For this review, take the finished solid that the model builds, in its own axes (mm). Face numbers are marked on the shaded views. A direction names the side the tool comes from. Give positions to 0.01 mm unless a question says otherwise; leave off trailing zeros. Loops run counter-clockwise (first coordinate to the right, second up) from the corner with the lowest first, then second, coordinate; pieces in that order, holes last. Notation, with made-up numbers: (-33, 58) - (-9, 58) arc R8 ccw to (-9, 70) - close; hole circle Ø2 at (-7, 53). An arc over 180 degrees is marked (long way). Answer as CSV lines item,"result".
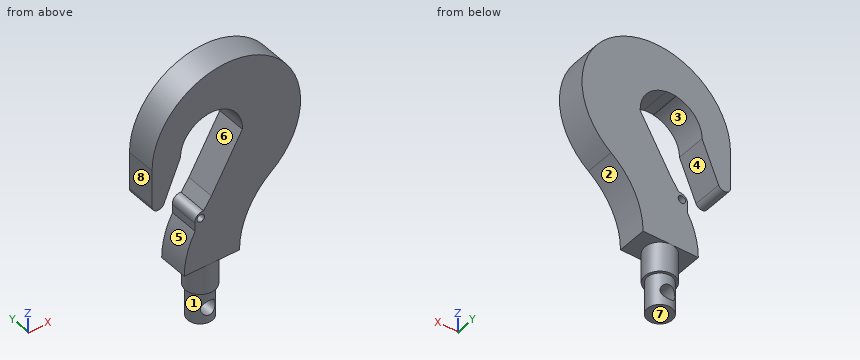
from build123d import *

# Parameters (mm, degrees)
F3_DEPTH = 60
F4_R     = 30
F5_DEPTH = 112
F6_R     = 15
F7_DEPTH = 163


with BuildPart() as f2:
    # F1 (on Front) → F2 (revolve)
    with BuildSketch(Plane.XZ):
        Polygon((-50, -120), (-50, -250), (0, -250), (0, 0), (-60, 0), (-60, -120), align=None)
    revolve(axis=Axis((0, 0, -125), (0, 0, -1)))

    # F0 (on Front) → F3 (join, symmetric)
    with BuildSketch(Plane.XZ):
        with BuildLine():
            ThreePointArc((113.275358, 0), (147.343032, 146.027594), (242.512075, 261.904762))
            ThreePointArc((242.512075, 261.904762), (192.752359, 769.029387), (-240, 500))
            Line((-240, 500), (-125, 500))
            ThreePointArc((-125, 500), (-95.197164, 581.009259), (-20, 623.389627))
            Line((-20, 623.389627), (-20, 624.947867))
            Line((-20, 624.947867), (20, 624.947867))
            Line((20, 624.947867), (20, 623.389627))
            ThreePointArc((20, 623.389627), (97.236318, 578.549974), (124.836727, 493.613169))
            Line((124.836727, 493.613169), (0, 278.411619))
            Line((0, 278.411619), (-31.669397, 232.573897))
            ThreePointArc((-31.669397, 232.573897), (-58.197727, 223.86417), (-66.061109, 197.072774))
            Line((-66.061109, 197.072774), (-66.061109, 164.52672))
            ThreePointArc((-66.061109, 164.52672), (-98.826102, 85.146444), (-110, 0))
            Line((-110, 0), (113.275358, 0))
        make_face()
        with BuildLine():
            Line((-125, 500), (-240, 500))
            Line((-240, 500), (-240, 350))
            ThreePointArc((-240, 350), (-219.930134, 325.490945), (-191.944498, 340.333365))
            Line((-191.944498, 340.333365), (-125, 500))
        make_face()
    extrude(amount=F3_DEPTH, both=True)

    # F4 (on Front) → F5 (cut, symmetric)
    with BuildSketch(Plane.XZ):
        with Locations((0, -190)):
            Circle(F4_R)
    extrude(amount=F5_DEPTH, both=True, mode=Mode.SUBTRACT)

    # F6 (on face) → F7 (cut, symmetric)
    with BuildSketch(Plane.XZ.offset(60)):
        with Locations((-43.483209, 207.776994)):
            Circle(F6_R)
    extrude(amount=F7_DEPTH, both=True, mode=Mode.SUBTRACT)


solid = f2.part
1) Machinability: for the marked faces 1, 2, 3, 4 and 5, which of the approach directions +Z, -Z, +X, -X, +Y, -Y give a long, thin tool a straight path to every point of the face, cutting with its end or side? Answer none if there is none.
From the geometry:
face 1,"-Z"
face 2,"-Z, +X, +Y, -Y"
face 3,"+Y, -Y"
face 4,"-Z, +Y, -Y"
face 5,"-X, +Y, -Y"
2) Wall thickness on line 1 (X direction, y = 1, z = -190); line 2 (X direction, y = 3, z = -190); line 3 (Z direction, x = 13, y = 1): over which ranges is each line inside the solid? List them lowest first. Write a range as from..to.
From the geometry:
line 1,"x = -49.99..-30, 30..49.99"
line 2,"x = -49.91..-30, 30..49.91"
line 3,"z = -250..-217.04, -162.96..300.82, 624.95..796.3"
3) Draft analysis for pull direction Z (two halves, no side actions). For the marked faces 6, 7 and 8, state which applies: pulls with the +Z half, pulls with the -Z half, needs draft (parallel to the pull), parting line crosses it, or undercut.
From the geometry:
face 6,"undercut"
face 7,"pulls with the -Z half"
face 8,"needs draft"
4) Consider section D-D on x = 198. Write out the cut boundary in (y, z), and give its area (3 significant figures).
From the geometry:
outline,"(-60, 220.77) - (60, 220.77) - (60, 766.38) - (-60, 766.38) - close"
area,"65,500 mm^2"
5) Insertion check: P1, Ø24, axis at x = -43.48, z = 207.78, coming from the +Y side; P2, Ø1.5, axis at x = 19, y = -3.5, coming from the +Z side; P3, Ø1.2, axis at y = 24.5, z = 624.5, coming from the +X side; P4, Ø1.5, axis at y = 12.5, z = 76.5, coming from the -X side. Each pin has a flat end and moves straight along its axis. Give the tip position at first contact, or say it passes through.
From the geometry:
P1,"passes through"
P2,"stops at z = 797.29"
P3,"stops at x = 333.22"
P4,"stops at x = -101.19"
6) Consider section B-B on y = 0. Write out the cut boundary in (x, z).
From the geometry:
outline,"(-240, 350) arc R25 ccw to (-191.94, 340.33) - (-125, 500) arc R125 cw to (-20, 623.39) - (-20, 624.95) - (20, 624.95) - (20, 623.39) arc R125 cw to (124.84, 493.61) - (0, 278.41) - (-31.67, 232.57) arc R30 ccw to (-66.06, 197.07) - (-66.06, 164.53) arc R330 ccw to (-110, 0) - (-60, 0) - (-60, -120) - (-50, -120) - (-50, -250) - (50, -250) - (50, -120) - (60, -120) - (60, 0) - (113.28, 0) arc R330 cw to (242.51, 261.9) arc R300 ccw (long way) to (-240, 500) - close; hole circle Ø30 at (-43.48, 207.78); hole circle Ø60 at (0, -190)"
7) Consider section A-A on z = 389. Write out the cut boundary in (x, y).
From the geometry:
outline,"(-240, -60) - (-171.54, -60) - (-171.54, 60) - (-240, 60) - close; (64.15, -60) - (338.71, -60) - (338.71, 60) - (64.15, 60) - close"
8) Consider section C-C on z = -190. Write out the cut boundary in (x, y).
From the geometry:
outline,"(-30, -40) - (-30, 40) arc R50 ccw to start; (30, -40) arc R50 ccw to (30, 40) - close"
